from build123d import *

# Parameters (mm, degrees)
PROFILEEXTRUDE_DEPTH = 73.76
HOSEWINDOW_W         = 16.29
HOSEWINDOW_H         = 11.5
HOSEWINDOWCUT_DEPTH  = 28
CAGESCREWS_R         = 2.4
CAGESCREWSCUT_DEPTH  = 28
AXLEHOLECUT_DEPTH    = 28
SETSCREWS_R          = 2.426338021
SETSCREWS_R_2        = 2.788762315
SETSCREWSCUT_DEPTH   = 28
FILLET1_R            = 1


with BuildPart() as part:
    # Profile → ProfileExtrude (new body)
    with BuildSketch(Plane.XY):
        with BuildLine():
            Line((-6.01073477, -43.62791746), (-6.01073477, -33.62791746))
            Line((-6.01073477, -33.62791746), (4.13926523, -33.62791746))
            Line((4.13926523, -33.62791746), (4.13926523, -18.13791746))
            ThreePointArc((4.13926523, -18.13791746), (7.563334043, -14.326029686), (9.63126523, -9.63791746))
            Line((9.63126523, -9.63791746), (11.94926523, -9.63791746))
            Line((11.94926523, -9.63791746), (11.94926523, 0.36208254))
            Line((11.94926523, 0.36208254), (9.35926523, 0.36208254))
            ThreePointArc((9.35926523, 0.36208254), (7.493178347, 4.320032013), (4.63926523, 7.63708254))
            Line((4.63926523, 7.63708254), (4.63926523, 17.41208254))
            Line((4.63926523, 17.41208254), (-6.51073477, 17.41208254))
            Line((-6.51073477, 17.41208254), (-6.51073477, 27.41208254))
            Line((-6.51073477, 27.41208254), (20.48926523, 27.41208254))
            Line((20.48926523, 27.41208254), (20.48926523, -43.62791746))
            Line((20.48926523, -43.62791746), (-6.01073477, -43.62791746))
        make_face()
    extrude(amount=PROFILEEXTRUDE_DEPTH)

    # HoseWindow → HoseWindowCut (cut, through all)
    with BuildSketch(Plane(origin=(20.48926523, 0, 0), x_dir=(0, 0, -1), z_dir=(1, 0, 0))):
        with Locations((-56.725, -37.87791746)):
            Rectangle(HOSEWINDOW_W, HOSEWINDOW_H)
    extrude(amount=-HOSEWINDOWCUT_DEPTH, mode=Mode.SUBTRACT)

    # CageScrews → CageScrewsCut (cut, through all)
    with BuildSketch(Plane(origin=(20.48926523, 0, 0), x_dir=(0, 0, -1), z_dir=(1, 0, 0))):
        with Locations((-66.26, 22.41208254)):
            Circle(CAGESCREWS_R)
        with Locations((-7.5, 22.41208254)):
            Circle(CAGESCREWS_R)
        with Locations((-7.5, -38.62791746)):
            Circle(CAGESCREWS_R)
        with Locations((-69.31, -38.62791746)):
            Circle(CAGESCREWS_R)
    extrude(amount=-CAGESCREWSCUT_DEPTH, mode=Mode.SUBTRACT)

    # AxleHole → AxleHoleCut (cut, through all)
    with BuildSketch(Plane(origin=(20.48926523, 0, 0), x_dir=(0, 0, -1), z_dir=(1, 0, 0))):
        with BuildLine():
            Line((-44.699, 2.307293484), (-47.361, 2.307293484))
            Line((-47.361, 2.307293484), (-47.361, 3.926293484))
            ThreePointArc((-47.361, 3.926293484), (-46.03, -9.21691746), (-44.699, 3.926293484))
            Line((-44.699, 3.926293484), (-44.699, 2.307293484))
        make_face()
    extrude(amount=-AXLEHOLECUT_DEPTH, mode=Mode.SUBTRACT)

    # SetScrews → SetScrewsCut (cut, through all)
    with BuildSketch(Plane(origin=(20.48926523, 0, 0), x_dir=(0, 0, -1), z_dir=(1, 0, 0))):
        with Locations((-68.03, -2.57791746)):
            Circle(SETSCREWS_R)
        with Locations((-6.03, -2.57791746)):
            Circle(SETSCREWS_R_2)
    extrude(amount=-SETSCREWSCUT_DEPTH, mode=Mode.SUBTRACT)

    # Fillet1
    fillet1_edges = [part.edges().sort_by_distance(p)[0] for p in [
        (20.48926523, -8.10791746, 0),
        (20.48926523, -43.62791746, 69.315),
        (20.48926523, 27.41208254, 36.88),
        (20.48926523, -8.10791746, 73.76),
        (20.48926523, -43.62791746, 24.29),
        (20.48926523, -37.87791746, 64.87),
        (20.48926523, -37.87791746, 48.58),
        (20.48926523, -32.12791746, 56.725),
    ]]
    fillet(fillet1_edges, radius=FILLET1_R)


solid = part.part
Geometry check sheet. Reference: the model listing, model coordinates, mm. A direction names the side the tool comes from. Round coordinates to 2 decimals unless told otherwise and drop trailing zeros. Loops run counter-clockwise (first coordinate to the right, second up) from the corner with the lowest first, then second, coordinate; pieces in that order, holes last.
Item 1: Cross-section at A-A on z = 46.03. Record the boundary of the cut face in (x, y).
Item 2: Access from +Z, -Z, +X, -X, +Y, -Y to the whole of each face (thin tool, end or side, straight path). Record for faces 1 (the flat face through (-6.011, -39, 24)), 2 (the cylindrical face through (7.18, 20.07, 8.02)), 3 (the flat face through (7, -38, 64.87)), 4 (the flat face through (11.949, -5, 36)).
Item 3: Thickness scan on line 1 (Y direction, x = 3.25, z = 7.5); line 2 (Y direction, x = 3, z = 66); line 3 (Z direction, x = 14.25, y = -34). Record the ranges inside material, lowest first.
Item 4: Cross-section at D-D on y = -7. Record the boundary of the cut face in (x, z).
Item 5: Gauge pin test, flat ends, axial feed: pin 1 (1 mm diameter, centred on y = -0.5, z = 38.5, fed in from -X); pin 2 (2.5 mm diameter, centred on y = -41, z = 70.5, fed in from -X); pin 3 (11 mm diameter, centred on y = -4.5, z = 24.5, fed in from -X). Record the tip position at first contact, or that the pin passes through.
Item 6: Cross-section at B-B on x = 2.75. Record the boundary of the cut face in (y, z).
Item 7: Cross-section at C-C on z = 17.5. Record the boundary of the cut face in (x, y).
Item 8: Mould release check, pull along Y, two halves, no side actions. Record for faces 5 (the cylindrical face through (7.425, -38.522, 71.708)), 6 (the flat face through (7, -43.628, 24)), 7 (the flat face through (20.489, -8, 36)): pulls with the +Y half, pulls with the -Y half, needs draft (parallel to the pull), parting line crosses it, or undercut.
Answer sheet:
1. outline: (-6.51, 17.41) - (4.64, 17.41) - (4.64, 7.64) arc R16.26 cw to (8.61, 2.31) - (20.49, 2.31) - (20.49, 26.41) arc R1 ccw to (19.49, 27.41) - (-6.51, 27.41) - close; (-6.01, -43.63) - (19.49, -43.63) arc R1 ccw to (20.49, -42.63) - (20.49, -9.22) - (11.95, -9.22) - (11.95, -9.64) - (9.63, -9.64) arc R16.26 cw to (4.14, -18.14) - (4.14, -33.63) - (-6.01, -33.63) - close
2. face 1: +Z, -Z, -X, -Y
2. face 2: +X, -X
2. face 3: +X, -X, -Y
2. face 4: +Z, -Z, -X
3. line 1: y = -43.63 to -41.03, -36.23 to -33.63, 17.41 to 20.01, 24.81 to 27.41
3. line 2: y = -43.63 to -33.63, 17.41 to 20.03, 24.8 to 27.41
3. line 3: z = 0 to 48.58, 64.87 to 73.76
4. outline: (11.95, 0) - (19.49, 0) arc R1 ccw to (20.49, 1) - (20.49, 41.08) - (11.95, 41.08) - close; (11.95, 50.98) - (20.49, 50.98) - (20.49, 72.76) arc R1 ccw to (19.49, 73.76) - (11.95, 73.76) - close
5. pin 1: stops at x = 11.95
5. pin 2: stops at x = -6.01
5. pin 3: stops at x = 9.14
6. outline: (-43.63, 0) - (-33.63, 0) - (-33.63, 48.58) - (-43.63, 48.58) - close; (-43.63, 64.87) - (-33.63, 64.87) - (-33.63, 73.76) - (-43.63, 73.76) - close; (17.41, 0) - (27.41, 0) - (27.41, 73.76) - (17.41, 73.76) - close; hole circle Ø4.8 at (-38.63, 7.5); hole circle Ø4.8 at (-38.63, 69.31); hole circle Ø4.8 at (22.41, 7.5); hole circle Ø4.8 at (22.41, 66.26)
7. outline: (-6.51, 17.41) - (4.64, 17.41) - (4.64, 7.64) arc R16.26 cw to (9.36, 0.36) - (11.95, 0.36) - (11.95, -9.64) - (9.63, -9.64) arc R16.26 cw to (4.14, -18.14) - (4.14, -33.63) - (-6.01, -33.63) - (-6.01, -43.63) - (19.49, -43.63) arc R1 ccw to (20.49, -42.63) - (20.49, 26.41) arc R1 ccw to (19.49, 27.41) - (-6.51, 27.41) - close
8. face 5: undercut
8. face 6: pulls with the -Y half
8. face 7: needs draft
